Input: part model. Units: mm. Frame: model coordinates. A direction names the side the tool comes from. Coordinates: 2 decimals unless noted, no trailing zeros. Loops run counter-clockwise (first coordinate to the right, second up) from the corner with the lowest first, then second, coordinate; pieces in that order, holes last.
Item 1: Reachability of faces 1 (the flat face through (-1, 10, -296)), 2 (the flat face through (-1, 10, 296)), 3 (the flat face through (-1, -10, -296)), 4 (the conical face through (623.622, -30.305, -23.237)), 5 (the flat face through (-1, -10, 296)) from +Z, -Z, +X, -X, +Y, -Y: full face, straight path, thin tool, end or side. Return the list, or none.
Item 2: Section A-A on x = -63. Return loops of the section in (y, z).
Item 3: Section B-B on z = 146. Return loops of the section in (x, y).
Item 4: Ray query, line 1 along Y through (x, z) = (-52.5, -403); line 2 along Y through (x, z) = (-70, 5.5); line 3 along Z through (x, y) = (126.5, -2.5). Return the intervals inside material, ascending.
Item 5: Contact query for flat-ended pins moving along their axis: P1, Ø4, axis at y = 47.5, z = 2, coming from the -X side; P2, Ø6, axis at x = 173, z = 46, coming from the +Y side; P3, Ø2, axis at x = 4, z = 12.5, coming from the -Y side. Output: stop coordinate, or through.
Item 6: Section C-C on x = 326. Return loops of the section in (y, z).
```python
from build123d import *

# Parameters (mm, degrees)
SKETCH004_W  = 200
SKETCH004_H  = 20
PAD_DEPTH    = 400
SKETCH005_W  = 200
SKETCH005_H  = 20
PAD001_DEPTH = 400


with BuildPart() as part:
    # Sketch → Revolution (revolve)
    with BuildSketch(Plane.XY):
        with BuildLine():
            Line((-500, 0), (500, 0))
            Line((500, 0), (700, 0))
            Line((500, 100), (700, 0))
            Line((-500, 100), (500, 100))
            ThreePointArc((-500, 100), (-570.710678, 70.710678), (-600, 0))
            Line((-500, 0), (-600, 0))
        make_face()
    revolve(axis=Axis((0, 0, 0), (1, 0, 0)))

    # Sketch004 → Pad (new body)
    with BuildSketch(Plane.XY.offset(98)):
        Rectangle(SKETCH004_W, SKETCH004_H)
    extrude(amount=PAD_DEPTH)

    # Sketch005 → Pad001 (join)
    with BuildSketch(Plane.XY.offset(-98)):
        Rectangle(SKETCH005_W, SKETCH005_H)
    extrude(amount=-PAD001_DEPTH)


solid = part.part
```
Results found:
1. face 1: -Z, +X, -X, +Y
1. face 2: +Z, +X, -X, +Y
1. face 3: -Z, +X, -X, -Y
1. face 4: +X
1. face 5: +Z, +X, -X, -Y
2. outline: (-10, -498) - (10, -498) - (10, -99.5) arc R100 ccw to (10, 99.5) - (10, 498) - (-10, 498) - (-10, 99.5) arc R100 ccw to (-10, -99.5) - close
3. outline: (-100, -10) - (100, -10) - (100, 10) - (-100, 10) - close
4. line 1: y = -10 to 10
4. line 2: y = -99.85 to 99.85
4. line 3: z = -99.97 to 99.97
5. P1: stops at x = -589.03
5. P2: stops at y = 90.28
5. P3: stops at y = -99.34
6. outline: circle Ø200 at (0, 0)
